Geometry check sheet. Reference: drawing and pictorial views, mm from the part's lowest x, y, z. Coordinates: 2 decimals unless noted, no trailing zeros. Write each loop counter-clockwise with the first axis right and the second up, starting at its lowest first coordinate (ties: lowest second). Pieces come first, ordered by that corner, then holes. Notation, with made-up numbers: (-14.5, -7) - (42.5, -7) arc R18 ccw to (42.5, -2) - close; hole circle Ø2 at (48.5, -20.5). An arc over 180 degrees is marked (long way). Answer as a JSON object with one key per item and string values. Group by question number.
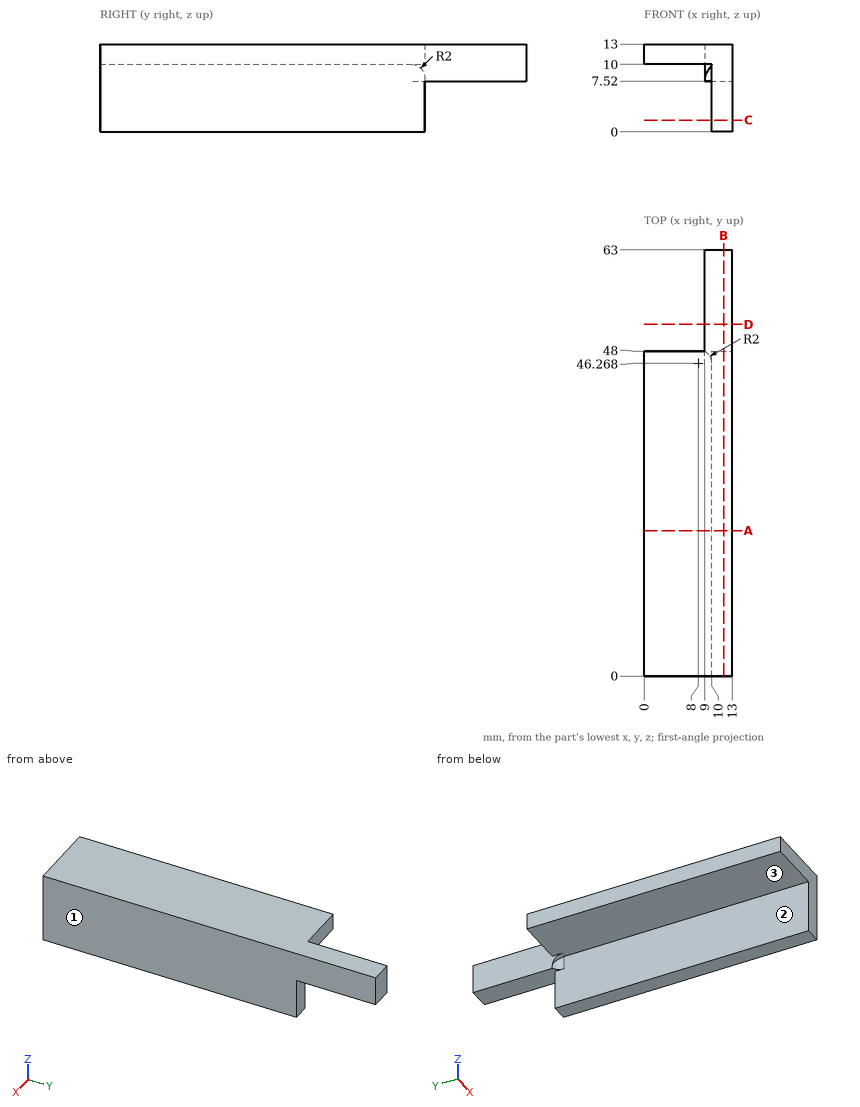
(1) Section check A-A (y = 21.5). Record the cut outline in (x, z).
(2) Draft check along X on the marked faces 1, 2 and 3. Enter one of: +X half, -X half, draft (parallel to the pull), parting line (faces both ways), or undercut.
(3) Section check D-D (y = 52). Record the cut outline in (x, z).
(4) Section check B-B (x = 11.75). Record the cut outline in (y, z).
(5) Section check C-C (z = 1.75). Record the cut outline in (x, y).
(6) Gauge pin test, flat ends, axial feed: pin 1 (3.5 mm diameter, centred on x = 11.5, z = 4, fed in from +Y); pin 2 (2 mm diameter, centred on x = 10.5, y = 56.5, fed in from -Z); pin 3 (3 mm diameter, centred on y = 17, z = 5, fed in from -X). Record the tip position at first contact, or that the pin passes through.
(7) Material ranges on L1, parallel to X at y = 51, z = 9.25; L2, parallel to X at y = 22, z = 8.5, recorded low to high. Write a range as [from, to].
Conclusion:
{
 "1": {"outline": "(0, 10) - (10, 10) - (10, 0) - (13, 0) - (13, 13) - (0, 13) - close"},
 "2": {"face 1": "+X half", "face 2": "-X half", "face 3": "draft"},
 "3": {"outline": "(9, 7.52) - (13, 7.52) - (13, 13) - (9, 13) - close"},
 "4": {"outline": "(0, 0) - (48, 0) - (48, 7.52) - (63, 7.52) - (63, 13) - (0, 13) - close"},
 "5": {"outline": "(10, 0) - (13, 0) - (13, 48) - (10, 48) - close"},
 "6": {"pin 1": "stops at y = 48", "pin 2": "stops at z = 7.52", "pin 3": "stops at x = 10"},
 "7": {"L1": "x = [9, 13]", "L2": "x = [10, 13]"}
}
